Design review of the part built by this model. Coordinates are the model's own, in mm. A direction names the side the tool comes from. Coordinates: 2 decimals unless noted, no trailing zeros. Write each loop counter-clockwise with the first axis right and the second up, starting at its lowest first coordinate (ties: lowest second). Pieces come first, ordered by that corner, then holes. Notation, with made-up numbers: M 66,48 L 85,48 A4 ccw 85,52 Z; hole C -9,69 d10. An arc over 180 degrees is marked long. Write item = value, one per line.
```python
from build123d import *

# Parameters (mm, degrees)
F0_W     = 20
F0_H     = 20
F1_DEPTH = 5
F3_DEPTH = 20
F4_W     = 20
F4_H     = 20
F5_DEPTH = 5


with BuildPart() as f1:
    # F0 (on Front) → F1 (new body)
    with BuildSketch(Plane.XZ):
        with Locations((10, 10)):
            Rectangle(F0_W, F0_H)
    extrude(amount=F1_DEPTH)

    # F2 (on face) → F3 (join)
    with BuildSketch(Plane.XZ.offset(5)):
        Polygon((0, 5), (0, 0), (20, 0), (20, 15), align=None)
    extrude(amount=F3_DEPTH)

    # F4 (on face) → F5 (join)
    with BuildSketch(Plane.XZ.offset(25)):
        with Locations((10, 10)):
            Rectangle(F4_W, F4_H)
    extrude(amount=F5_DEPTH)


solid = f1.part
```
Q1. For P1, Ø6, axis at y = -21.5, z = 11, coming from the -X side, flat-tipped, find the tip position at first contact; note if it passes through.
Check result:
P1 = 6
Q2. The part is to be moulded in two halves that separate along Y. For faces 1 (the flat face through (10, -15, 0)), 2 (the flat face through (10, -30, 10)), 3 (the flat face through (10, 0, 10)), 4 (the flat face through (8, -5, 14)), say which applies: +Y half, -Y half, draft (parallel to the pull), parting line (faces both ways), or undercut.
Check result:
face_1 = draft
face_2 = -Y half
face_3 = +Y half
face_4 = undercut
Q3. Consider section A-A, the plane z = 18. State the section outline as (x, y) points.
Check result:
outline = M 0,-30 L 20,-30 L 20,-25 L 0,-25 Z; M 0,-5 L 20,-5 L 20,0 L 0,0 Z
Q4. Wall thickness on line 1 (Y direction, x = 2.25, z = 18.75); line 2 (Z direction, x = 18, y = -15.75); line 3 (Z direction, x = 9, y = -18.25): over which ranges is each line inside the solid? List them lowest first.
Check result:
line_1 = -30 to -25, -5 to 0
line_2 = 0 to 14
line_3 = 0 to 9.5
Q5. Consider section D-D, the plane y = -6. State the section outline as (x, z) points, and give its area (3 significant figures).
Check result:
outline = M 0,0 L 20,0 L 20,15 L 0,5 Z
area = 200 mm²
Q6. Consider section C-C, the plane z = 13. State the section outline as (x, y) points.
Check result:
outline = M 0,-30 L 20,-30 L 20,0 L 0,0 L 0,-5 L 16,-5 L 16,-25 L 0,-25 Z
Q7. Machinability: for faces 5 (the flat face through (20, -15, 8)), 6 (the flat face through (8, -25, 14)), which of the approach directions +Z, -Z, +X, -X, +Y, -Y give a long, thin tool a straight path to every point of the face, cutting with its end or side? Answer none if there is none.
Check result:
face_5 = +Z, -Z, +X, +Y, -Y
face_6 = +Z, -X
Q8. Consider section B-B, the plane x = 12. State the section outline as (y, z) points.
Check result:
outline = M -30,0 L 0,0 L 0,20 L -5,20 L -5,11 L -25,11 L -25,20 L -30,20 Z
